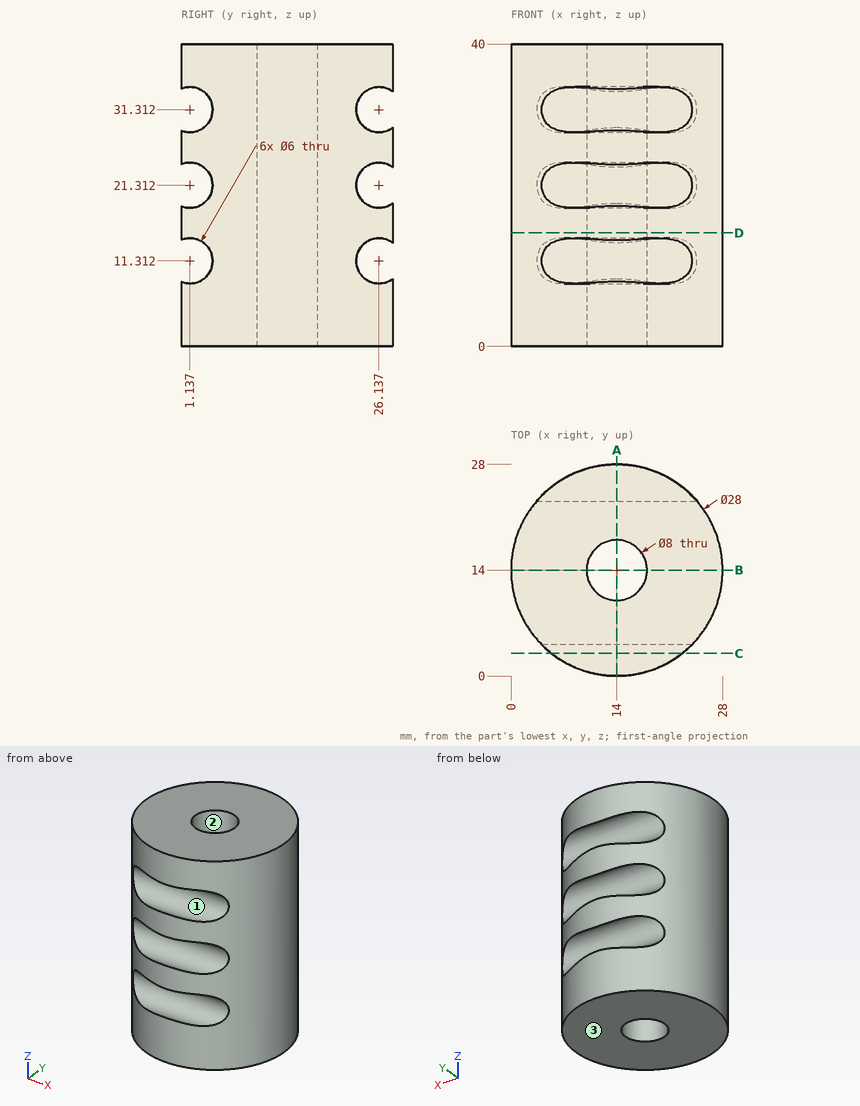
Could you check a few things on this drawing? It's one solid part, dimensions in mm from its lowest x, y, z. Coordinates: 2 decimals unless noted, no trailing zeros. Order: outer loops, then holes, each group sorted by start corner. A loop starts at its lowest first (then second) coordinate and runs counter-clockwise, first axis right, second up. Notation, with made-up numbers: M 2,-26.75 L 52,-26.75 A11 cw 52,-22.75 Z; hole C -6.5,30 d4. An arc over 180 degrees is marked long. Use one line per item in the form item = value. Start each with the question number.
1. Suppose I cut it at A-A on x = 14. Write out the boundary of the cut face in (y, z), then the cut area to 3 significant figures.
2. Suppose I cut it at D-D on z = 15. Write out the boundary of the cut face in (x, y).
3. Suppose I cut it at B-B on y = 14. Write out the boundary of the cut face in (x, z).
4. Suppose I cut it at C-C on y = 3. Write out the boundary of the cut face in (x, z).
5. We'd pull the mould along Z, two halves only. Please class the marked faces 1, 2 and 3: +Z half, -Z half, draft (parallel to the pull), parting line (faces both ways), or undercut.
6. Please list where these lines run through material, in increasing order: line 1 (X direction, y = 14.25, z = 2.5); line 2 (Y direction, x = 14, z = 18); line 3 (X direction, y = 12.25, z = 17).
7. For pin 1 (1 mm diameter, centred on y = 15, z = 24, fed in from +X); pin 2 (3.5 mm diameter, centred on y = 1.14, z = 31.31, fed in from -X); pin 3 (7 mm diameter, centred on y = 26.14, z = 31.31, fed in from +X) (1 decimal); pin 4 (6 mm diameter, centred on x = 17.5, z = 32, fed in from -Y), each with a flat end and sliding along its axis, tell me the tip position at first contact or that it passes through.
Geometry says:
q1.outline = M 0,0 L 10,0 L 10,40 L 0,40 L 0,34.09 A3 cw long 0,28.54 L 0,24.09 A3 cw long 0,18.54 L 0,14.09 A3 cw long 0,8.54 Z; M 18,0 L 28,0 L 28,8.96 A3 cw long 28,13.66 L 28,18.96 A3 cw long 28,23.66 L 28,28.96 A3 cw long 28,33.66 L 28,40 L 18,40 Z
q1.area = 664 mm^2
q2.outline = C 14,14 d28; hole C 14,14 d8
q3.outline = M 0,0 L 10,0 L 10,40 L 0,40 Z; M 18,0 L 28,0 L 28,40 L 18,40 Z
q4.outline = M 5.34,0 L 22.66,0 L 22.66,8.96 L 5.34,8.96 Z; M 5.34,13.66 L 22.66,13.66 L 22.66,18.96 L 5.34,18.96 Z; M 5.34,23.66 L 22.66,23.66 L 22.66,28.96 L 5.34,28.96 Z; M 5.34,33.66 L 22.66,33.66 L 22.66,40 L 5.34,40 Z
q5.face_1 = undercut
q5.face_2 = draft
q5.face_3 = -Z half
q6.line_1 = 0 to 10.01, 17.99 to 28
q6.line_2 = 0 to 10, 18 to 28
q6.line_3 = 0.11 to 10.4, 17.6 to 27.89
q7.pin_1 = 27.99
q7.pin_2 = through
q7.pin_3 = 25
q7.pin_4 = 0.07
